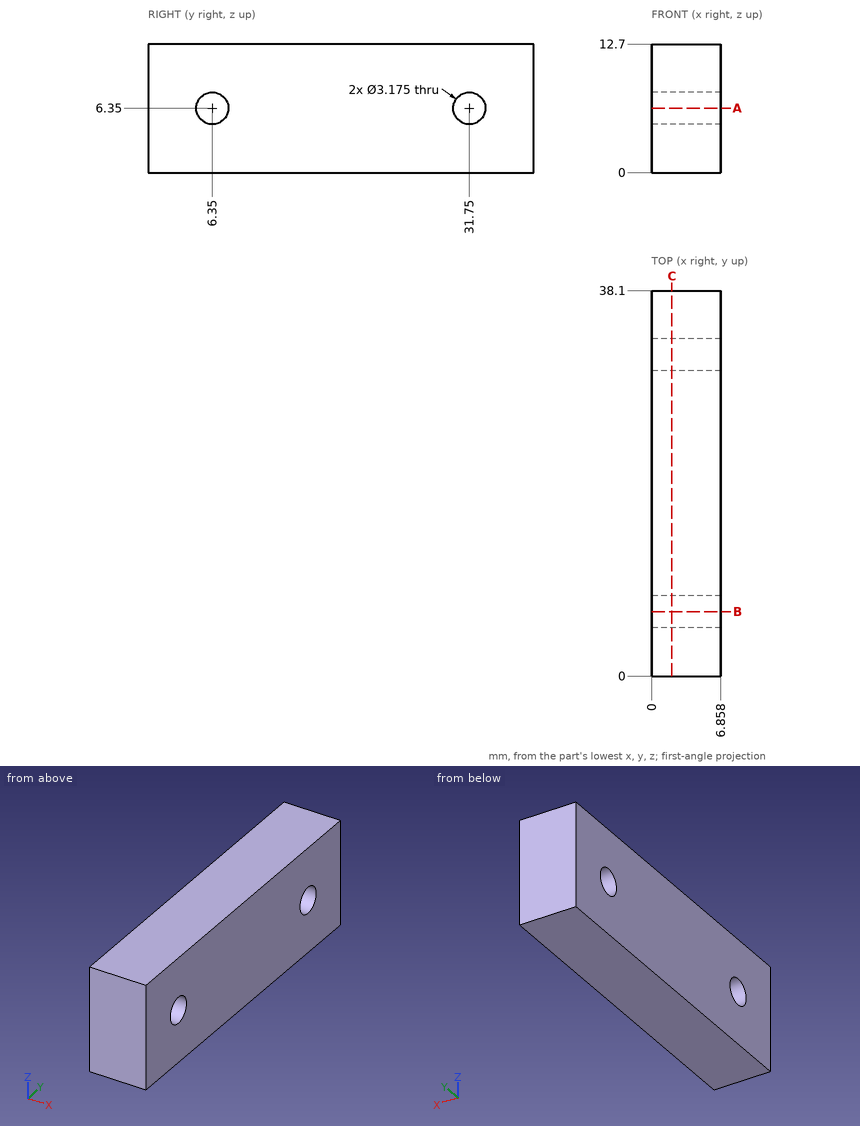
Design review of the part shown in the three views and the two pictorial views. Dimensions are in mm from the part's minimum x, y and z. Round coordinates to 2 decimals unless told otherwise and drop trailing zeros. Loops run counter-clockwise (first coordinate to the right, second up) from the corner with the lowest first, then second, coordinate; pieces in that order, holes last. Notation, with made-up numbers: (-19.75, 67) - (-4.75, 67) arc R24 cw to (-4.75, 81) - close; hole circle Ø1 at (40, 40). An arc over 180 degrees is marked (long way). One line per item, written item: value. Start each with the question number.
Item 1: Take a section at C-C (x = 2). State how many separate pieces and enclosed holes the cut face has, plus the area to 3 significant figures.
Item 2: Clearance check with a flat-ended pin moving along its axis: pin 1 Ø2.5 at (y, z) = (6.35, 6.35) entering from +X. State where the tip first meets the part, or that it passes through.
Item 3: Take a section at B-B (y = 6.35). Give the boundary of the cut face in (x, z).
Item 4: For L1, parallel to Z at x = 3, y = 31.75; L2, parallel to Y at x = 1.75, z = 6.35; L3, parallel to Y at x = 2.25, z = 7.75, list the stretches that pass through material, from the lowest coordinate up.
Item 5: Take a section at A-A (z = 6.35). Give the boundary of the cut face in (x, y).
Answer below:
1. separate pieces: 1
1. enclosed holes: 2
1. area: 468 mm2
2. pin 1: passes through
3. outline: (0, 0) - (6.86, 0) - (6.86, 4.76) - (0, 4.76) - close; (0, 7.94) - (6.86, 7.94) - (6.86, 12.7) - (0, 12.7) - close
4. L1: z = 0 to 4.76, 7.94 to 12.7
4. L2: y = 0 to 4.76, 7.94 to 30.16, 33.34 to 38.1
4. L3: y = 0 to 5.6, 7.1 to 31, 32.5 to 38.1
5. outline: (0, 0) - (6.86, 0) - (6.86, 4.76) - (0, 4.76) - close; (0, 7.94) - (6.86, 7.94) - (6.86, 30.16) - (0, 30.16) - close; (0, 33.34) - (6.86, 33.34) - (6.86, 38.1) - (0, 38.1) - close
